Design review of the part shown in the three views and the two pictorial views. Dimensions are in mm from the part's minimum x, y and z. Round coordinates to 2 decimals unless told otherwise and drop trailing zeros. Write each loop counter-clockwise with the first axis right and the second up, starting at its lowest first coordinate (ties: lowest second). Pieces come first, ordered by that corner, then holes. Notation, with made-up numbers: (6, 71) -> (16, 71) arc R19 cw to (16, 84) -> close; hole circle Ø3 at (23.25, 19.5). An arc over 180 degrees is marked (long way). One line per question, with ' | ' between items. Start each with the question number.
1) Consider section C-C (y = 5). Give the boundary of the cut face in (x, z).
2) Consider section A-A (x = 17.5). Give the boundary of the cut face in (y, z), then the cut area to 3 significant figures.
3) Consider section B-B (z = 3.4). Give the boundary of the cut face in (x, y).
4) For probe 1 along Y at (x, z) = (4.75, 1.35); probe 2 along Y at (x, z) = (30.25, 3.25); probe 3 along X at (y, z) = (14.75, 0.85), list the stretches that pass through material, from the lowest coordinate up.
5) Consider section D-D (y = 40.25). Give the boundary of the cut face in (x, z).
6) Insertion check: pin 1 Ø5 at (x, y) = (30.25, 40.25) entering from +Z. The pin has a flat end and moves straight along its axis. Give the tip position at first contact, or say it passes through.
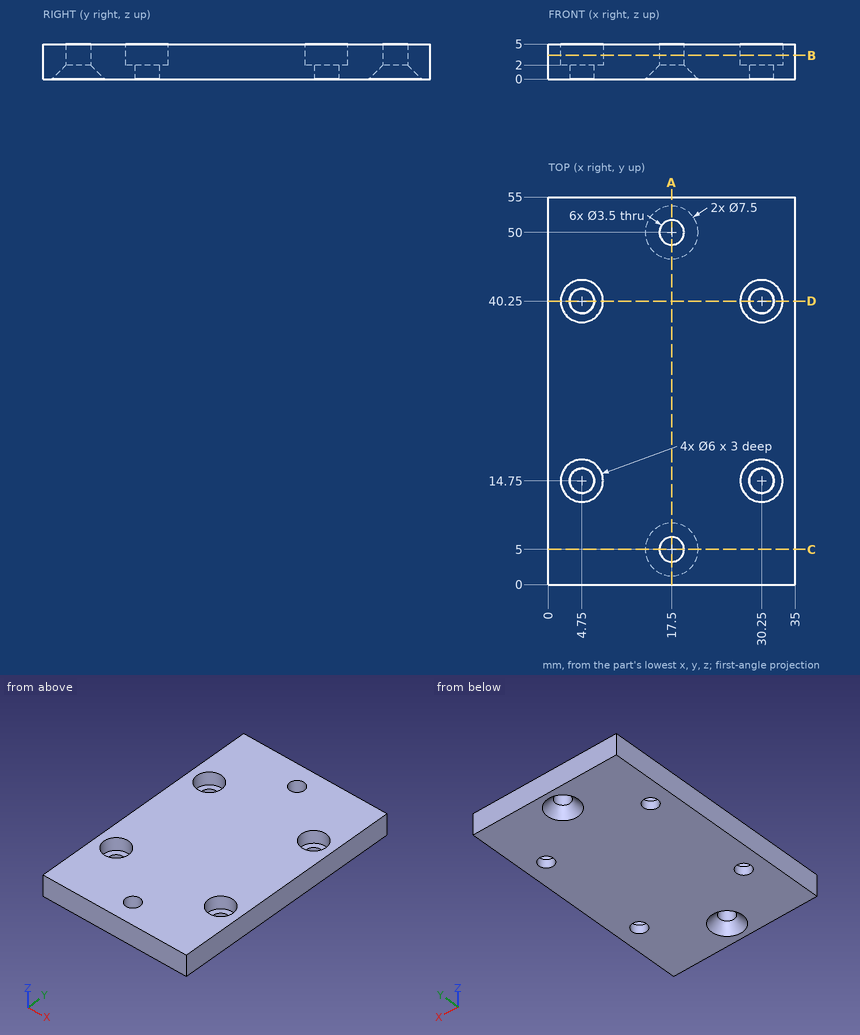
From the geometry:
1) outline: (0, 0) -> (13.75, 0) -> (15.75, 2) -> (15.75, 5) -> (0, 5) -> close; (19.25, 2) -> (21.25, 0) -> (35, 0) -> (35, 5) -> (19.25, 5) -> close
2) outline: (0, 0) -> (1.25, 0) -> (3.25, 2) -> (3.25, 5) -> (0, 5) -> close; (6.75, 2) -> (8.75, 0) -> (46.25, 0) -> (48.25, 2) -> (48.25, 5) -> (6.75, 5) -> close; (51.75, 2) -> (53.75, 0) -> (55, 0) -> (55, 5) -> (51.75, 5) -> close | area: 232 mm2
3) outline: (0, 0) -> (35, 0) -> (35, 55) -> (0, 55) -> close; hole circle Ø6 at (4.75, 14.75); hole circle Ø6 at (4.75, 40.25); hole circle Ø3.5 at (17.5, 5); hole circle Ø3.5 at (17.5, 50); hole circle Ø6 at (30.25, 14.75); hole circle Ø6 at (30.25, 40.25)
4) probe 1: y = 0 to 13, 16.5 to 38.5, 42 to 55 | probe 2: y = 0 to 11.75, 17.75 to 37.25, 43.25 to 55 | probe 3: x = 0 to 3, 6.5 to 28.5, 32 to 35
5) outline: (0, 0) -> (3, 0) -> (3, 2) -> (1.75, 2) -> (1.75, 5) -> (0, 5) -> close; (6.5, 0) -> (28.5, 0) -> (28.5, 2) -> (27.25, 2) -> (27.25, 5) -> (7.75, 5) -> (7.75, 2) -> (6.5, 2) -> close; (32, 0) -> (35, 0) -> (35, 5) -> (33.25, 5) -> (33.25, 2) -> (32, 2) -> close
6) pin 1: stops at z = 2
